Read the model definition and answer for the solid it produces. Units are mm, in the model's axes. Coordinates: 2 decimals unless noted, no trailing zeros. Loops run counter-clockwise (first coordinate to the right, second up) from the corner with the lowest first, then second, coordinate; pieces in that order, holes last. Notation, with made-up numbers: M -14,-25.5 L -5,-25.5 A32 cw -5,11.5 Z; hole C 16.5,-7 d9. An arc over 180 degrees is marked long. Use one line per item in the form item = value. Start each with the question number.
1. The part is cut by section B-B (x = -2). Give the vertices of the cut face in (y, z).
2. Flat-ended cylindrical pins translate along their axes: pin 1 (1.5 mm diameter, centred on x = 7, z = 141, fed in from +Y); pin 2 (3 mm diameter, centred on x = -6, z = 160, fed in from +Y); pin 3 (4 mm diameter, centred on y = 9, z = 135.5, fed in from -X); pin 4 (5.5 mm diameter, centred on x = 0, z = 190.5, fed in from -Y). Find the tip coordinate at first contact, or state that the pin passes through.
3. The part is cut by section A-A (y = 0). Give the vertices of the cut face in (x, z) (1 decimal).
4. Find the intervals of material crossed by probe 1 along Z at (x, y) = (1.5, -0.5); probe 2 along X at (y, z) = (11, 139.7); probe 3 along X at (y, z) = (7, 142), in increasing order. Write a range as [from, to].
5. The part is cut by section C-C (z = 39). Give the vertices of the cut face in (x, y) (3 decimals).
from build123d import *

# Parameters (mm, degrees)
SKETCH1_R               = 22.225
BOSS_EXTRUDE1_DEPTH     = 203.2
CUT_EXTRUDE1_DEPTH      = 203.2
CUT_EXTRUDE1_DEPTH_BACK = 203.2
SKETCH2_R               = 4.7625


with BuildPart() as part:
    # Sketch1 → Boss-Extrude1 (new body)
    with BuildSketch(Plane.XY):
        Circle(SKETCH1_R)
    extrude(amount=BOSS_EXTRUDE1_DEPTH)

    # Sketch2 → Cut-Extrude1 (cut, two sides: drawn at the far end of the back side and taken through both)
    with BuildSketch(Plane(origin=(0, 0, 0), x_dir=(1, 0, 0), z_dir=(0, 1, 0)).offset(-CUT_EXTRUDE1_DEPTH_BACK)):
        with Locations(Location((0, -190.5, 0), (0, 0, 90))):
            Circle(SKETCH2_R)
        with Locations(Location((0, -139.7, 0), (0, 0, 90))):
            Circle(SKETCH2_R)
        with Locations(Location((0, -12.7, 0), (0, 0, 90))):
            Circle(SKETCH2_R)
        with Locations(Location((0, -63.5, 0), (0, 0, 90))):
            Circle(SKETCH2_R)
    extrude(amount=CUT_EXTRUDE1_DEPTH + CUT_EXTRUDE1_DEPTH_BACK, mode=Mode.SUBTRACT)


solid = part.part
Computed values:
q1.outline = M -22.13,0 L 22.13,0 L 22.13,8.38 L -22.13,8.38 Z; M -22.13,17.02 L 22.13,17.02 L 22.13,59.18 L -22.13,59.18 Z; M -22.13,67.82 L 22.13,67.82 L 22.13,135.38 L -22.13,135.38 Z; M -22.13,144.02 L 22.13,144.02 L 22.13,186.18 L -22.13,186.18 Z; M -22.13,194.82 L 22.13,194.82 L 22.13,203.2 L -22.13,203.2 Z
q2.pin_1 = 21.33
q2.pin_2 = 21.76
q2.pin_3 = -21.09
q2.pin_4 = through
q3.outline = M -22.2,0 L 22.2,0 L 22.2,203.2 L -22.2,203.2 Z; hole C 0,12.7 d9.5; hole C 0,63.5 d9.5; hole C 0,139.7 d9.5; hole C 0,190.5 d9.5
q4.probe_1 = [0, 8.18], [17.22, 58.98], [68.02, 135.18], [144.22, 185.98], [195.02, 203.2]
q4.probe_2 = [-19.31, -4.76], [4.76, 19.31]
q4.probe_3 = [-21.09, -4.17], [4.17, 21.09]
q5.outline = C 0,0 d44.45
